Could you check a few things on this model? Use its own coordinates, in mm. Give positions to 0.01 mm unless a question says otherwise; leave off trailing zeros. Order: outer loops, then holes, each group sorted by start corner. A loop starts at its lowest first (then second) coordinate and runs counter-clockwise, first axis right, second up. Notation, with made-up numbers: M 10,51 L 33,51 A30 ccw 33,75 Z; hole C 0,68.5 d6. An arc over 180 degrees is marked long. Return JSON: item names as keys, results as strings. Group by question number.
```python
from build123d import *

# Parameters (mm, degrees)
ESBO_O1_W                = 50
ESBO_O1_H                = 25
ESBO_O1_R                = 4.25
ESBO_O1_R_2              = 1
RESSALTO_EXTRUS_O1_DEPTH = 3


with BuildPart() as part:
    # Esboço1 → Ressalto-extrusão1 (new body)
    with BuildSketch(Plane.XY):
        Rectangle(ESBO_O1_W, ESBO_O1_H)
        Circle(ESBO_O1_R, mode=Mode.SUBTRACT)
        with Locations((0, 8)):
            Circle(ESBO_O1_R_2, mode=Mode.SUBTRACT)
        with Locations((5.656854249, 5.656854249)):
            Circle(ESBO_O1_R_2, mode=Mode.SUBTRACT)
        with Locations((8, 0)):
            Circle(ESBO_O1_R_2, mode=Mode.SUBTRACT)
        with Locations((5.656854249, -5.656854249)):
            Circle(ESBO_O1_R_2, mode=Mode.SUBTRACT)
        with Locations((0, -8)):
            Circle(ESBO_O1_R_2, mode=Mode.SUBTRACT)
        with Locations((-5.656854249, -5.656854249)):
            Circle(ESBO_O1_R_2, mode=Mode.SUBTRACT)
        with Locations((-8, 0)):
            Circle(ESBO_O1_R_2, mode=Mode.SUBTRACT)
        with Locations((-5.656854249, 5.656854249)):
            Circle(ESBO_O1_R_2, mode=Mode.SUBTRACT)
        with Locations((-15, 8)):
            Circle(ESBO_O1_R_2, mode=Mode.SUBTRACT)
        with Locations((-15, -8)):
            Circle(ESBO_O1_R_2, mode=Mode.SUBTRACT)
        with Locations(Location((15, -8, 0), (0, 0, 180))):
            Circle(ESBO_O1_R_2, mode=Mode.SUBTRACT)
        with Locations(Location((15, 8, 0), (0, 0, 180))):
            Circle(ESBO_O1_R_2, mode=Mode.SUBTRACT)
        with Locations((23, 8)):
            Circle(ESBO_O1_R_2, mode=Mode.SUBTRACT)
        with Locations((23, -8)):
            Circle(ESBO_O1_R_2, mode=Mode.SUBTRACT)
        with Locations(Location((-23, -8, 0), (0, 0, 180))):
            Circle(ESBO_O1_R_2, mode=Mode.SUBTRACT)
        with Locations(Location((-23, 8, 0), (0, 0, 180))):
            Circle(ESBO_O1_R_2, mode=Mode.SUBTRACT)
    extrude(amount=RESSALTO_EXTRUS_O1_DEPTH)


solid = part.part
```
1. Imagine slicing it at A-A, the plane x = 0. Please give me the cut outline in (y, z), plus the area to 3 significant figures.
2. Imagine slicing it at B-B, the plane y = 0. Please give me the cut outline in (x, z).
3. Imagine slicing it at D-D, the plane z = 0.7. Count the separate pieces of the cut face and the enclosed holes in it, plus the area to 3 significant figures.
4. Imagine slicing it at C-C, the plane x = 8. Please give me the cut outline in (y, z).
5. If we mould it in two halves opening along Y, with no side actions, what happens to faces 1 (the flat face through (25, 0, 1)), 2 (the flat face through (0, -12.5, 1)), 3 (the cylindrical face through (-6.656, -5.613, 1.479))? For each: pulls with the +Y half, pulls with the -Y half, needs draft (parallel to the pull), parting line crosses it, or undercut.
6. I need wall thicknesses on L1, parallel to Y at x = -15, z = 0.8; L2, parallel to X at y = 5.75, z = 2.6; L3, parallel to X at y = 6, z = 0.6. Which ranges of each line are inside material? Lowest first, please. Write a range as from..to.
7. For pin 1 (4 mm diameter, centred on x = 0.5, y = 0.5, fed in from -Z), with a flat end and sliding along its axis, tell me the tip position at first contact or that it passes through.
Values:
{
 "1": {"outline": "M -12.5,0 L -9,0 L -9,3 L -12.5,3 Z; M -7,0 L -4.25,0 L -4.25,3 L -7,3 Z; M 4.25,0 L 7,0 L 7,3 L 4.25,3 Z; M 9,0 L 12.5,0 L 12.5,3 L 9,3 Z", "area": "37.5 mm²"},
 "2": {"outline": "M -25,0 L -9,0 L -9,3 L -25,3 Z; M -7,0 L -4.25,0 L -4.25,3 L -7,3 Z; M 4.25,0 L 7,0 L 7,3 L 4.25,3 Z; M 9,0 L 25,0 L 25,3 L 9,3 Z"},
 "3": {"separate pieces": "1", "enclosed holes": "17", "area": "1,140 mm²"},
 "4": {"outline": "M -12.5,0 L -1,0 L -1,3 L -12.5,3 Z; M 1,0 L 12.5,0 L 12.5,3 L 1,3 Z"},
 "5": {"face 1": "needs draft", "face 2": "pulls with the -Y half", "face 3": "undercut"},
 "6": {"L1": "y = -12.5..-9, -7..7, 9..12.5", "L2": "x = -25..-6.65, -4.66..4.66, 6.65..25", "L3": "x = -25..-6.6, -4.72..4.72, 6.6..25"},
 "7": {"pin 1": "passes through"}
}
